The model under review builds one solid part; all positions refer to its coordinate system, in mm. Face numbers are marked on the shaded views. Round coordinates to 2 decimals unless told otherwise and drop trailing zeros. Loops run counter-clockwise (first coordinate to the right, second up) from the corner with the lowest first, then second, coordinate; pieces in that order, holes last. Notation, with made-up numbers: (-4.5, -23) - (26.5, -23) arc R15 ccw to (26.5, -9) - close; hole circle Ø5 at (39, 15.25). An arc over 180 degrees is marked (long way). Answer as CSV lines item,"result".
from build123d import *

# Parameters (mm, degrees)
F0_W      = 38.3663107641
F0_H      = 42.2096475959
F1_DEPTH  = 0.6858
F3_W      = 400
F3_H      = 300.087749958
F4_DEPTH  = 5
F5_W      = 5
F5_H      = 300.087749958
F6_DEPTH  = 20
F7_W      = 5
F7_H      = 300.087749958
F8_DEPTH  = 20
F9_W      = 400
F9_H      = 25
F10_DEPTH = 5
F11_W     = 5
F11_H     = 300.087749958
F12_DEPTH = 20
F13_W     = 400
F13_H     = 25
F14_DEPTH = 5
F15_R     = 5
F16_DEPTH = 10
F17_R     = 7.5
F17_R_2   = 5
F18_DEPTH = 10


with BuildPart() as f1:
    # F0 (on Top) → F1 (new body)
    with BuildSketch(Plane.XY):
        with Locations((-14.0401979443, 21.1048237979)):
            Rectangle(F0_W, F0_H)
    extrude(amount=F1_DEPTH)


with BuildPart() as f4:
    # F3 (on Top) → F4 (new body)
    with BuildSketch(Plane.XY):
        Rectangle(F3_W, F3_H)
    extrude(amount=F4_DEPTH)

    # F5 (on face) → F6 (join)
    with BuildSketch(Plane.XY.offset(5)):
        with Locations((-197.5, 0)):
            Rectangle(F5_W, F5_H)
    extrude(amount=F6_DEPTH)

    # F7 (on face) → F8 (join)
    with BuildSketch(Plane.XY.offset(5)):
        with Locations((197.5, 0)):
            Rectangle(F7_W, F7_H)
    extrude(amount=F8_DEPTH)

    # F9 (on face) → F10 (join)
    with BuildSketch(Plane(origin=(0, 150.043874979, 0), x_dir=(-1, 0, 0), z_dir=(0, 1, 0))):
        with Locations((0, 12.5)):
            Rectangle(F9_W, F9_H)
    extrude(amount=F10_DEPTH)

    # F11 (on face) → F12 (join)
    with BuildSketch(Plane.XY.offset(5)):
        Rectangle(F11_W, F11_H)
    extrude(amount=F12_DEPTH)

    # F13 (on face) → F14 (join)
    with BuildSketch(Plane.XZ.offset(150.043874979)):
        with Locations((0, 12.5)):
            Rectangle(F13_W, F13_H)
    extrude(amount=F14_DEPTH)

    # F15 (on face) → F16 (join)
    with BuildSketch(Plane.XZ.offset(155.043874979)):
        with Locations((0, 12.090690434)):
            Circle(F15_R)
    extrude(amount=F16_DEPTH)

    # F17 (on face) → F18 (join)
    with BuildSketch(Plane.XZ.offset(165.043874979)):
        with Locations((0, 12.090690434)):
            Circle(F17_R)
        with Locations((0, 12.090690434)):
            Circle(F17_R_2, mode=Mode.SUBTRACT)
        with Locations((0, 12.090690434)):
            Circle(F17_R_2)
    extrude(amount=F18_DEPTH)


solid = f4.part
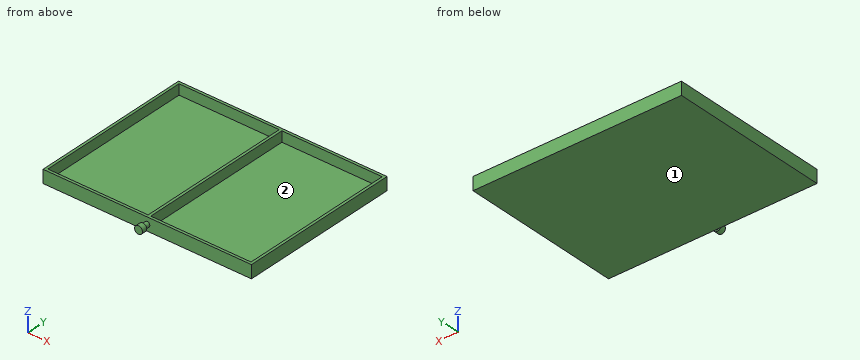
1. Wall thickness on probe 1 along X at (y, z) = (-130, 5.5); probe 2 along Y at (x, z) = (5.5, 15); probe 3 along Y at (x, z) = (-146.5, 13): over which ranges is each line inside the solid? List them lowest first.
Numbers:
probe 1,"x = -200 to -195, -2.5 to 2.5, 195 to 200"
probe 2,"y = -175.04 to -165.04, -155.04 to -150.04, 150.04 to 155.04"
probe 3,"y = -155.04 to -150.04, 150.04 to 155.04"
2. Take a section at A-A (x = -40.5). State the section outline as (y, z) points.
Numbers:
outline,"(-155.04, 0) - (155.04, 0) - (155.04, 25) - (150.04, 25) - (150.04, 5) - (-150.04, 5) - (-150.04, 25) - (-155.04, 25) - close"
3. Draft analysis for pull direction Y (two halves, no side actions). For the marked faces 1 and 2, state which applies: +Y half, -Y half, draft (parallel to the pull), parting line (faces both ways), or undercut.
Numbers:
face 1,"draft"
face 2,"undercut"
4. Take a section at B-B (y = 97.5). State the section outline as (x, z) points.
Numbers:
outline,"(-200, 0) - (200, 0) - (200, 25) - (195, 25) - (195, 5) - (2.5, 5) - (2.5, 25) - (-2.5, 25) - (-2.5, 5) - (-195, 5) - (-195, 25) - (-200, 25) - close"
5. Clearance check with flat-ended pins moving along their axes: pin 1 (1 mm diameter, centred on x = -31.5, z = 7, fed in from -Y); pin 2 (5 mm diameter, centred on x = 108, y = -89, fed in from -Z). State where each tip first meets the part, or that it passes through.
Numbers:
pin 1,"stops at y = -155.04"
pin 2,"stops at z = 0"
